Verification items for this drawing (mm, ordinates from the low corner). A direction names the side the tool comes from. Give positions to 0.01 mm unless a question says otherwise; leave off trailing zeros. Loops run counter-clockwise (first coordinate to the right, second up) from the corner with the lowest first, then second, coordinate; pieces in that order, holes last. Notation, with made-up numbers: (76.25, -4.75) -> (125.25, -4.75) arc R22 cw to (125.25, 4.25) -> close; hole circle Ø9 at (5, -32). An arc over 180 degrees is marked (long way). Answer in a Markdown table with one row per item. Add a question column.
Q1. Gauge pin test, flat ends, axial feed: P1, Ø3, axis at y = 6.5, z = 9.5, coming from the -X side; P2, Ø4, axis at x = 5, z = 15.5, coming from the +Y side; P3, Ø4.5, axis at x = 2, y = 5, coming from the -Z side. Record the tip position at first contact, or that the pin passes through.
Q2. Section check A-A on x = 2. Enter the section's corners in (y, z).
Q3. Set-up check for the marked faces 5, 6, 7 and 8: record each of +Z, -Z, +X, -X, +Y, -Y from which the full face is reachable in a straight line by a thin tool's end or side.
Q4. Section check B-B on z = 25.25. Enter the section's corners in (x, y).
Q5. Material ranges on probe 1 along Y at (x, z) = (10, 7); probe 2 along Z at (x, y) = (2.25, 2.5); probe 3 along Z at (x, y) = (11.5, 9.05), recorded low to high.
Q6. Release check for a two-part mould opening along X. For the marked faces 1, 2, 3 and 4 record: pulls with the +X half, pulls with the -X half, needs draft (parallel to the pull), parting line crosses it, or undercut.
Q7. Section check C-C on z = 4. Enter the section's corners in (x, y), and give its area (3 significant figures).
Q8. Section check D-D on x = 5.5. Enter the section's corners in (y, z).
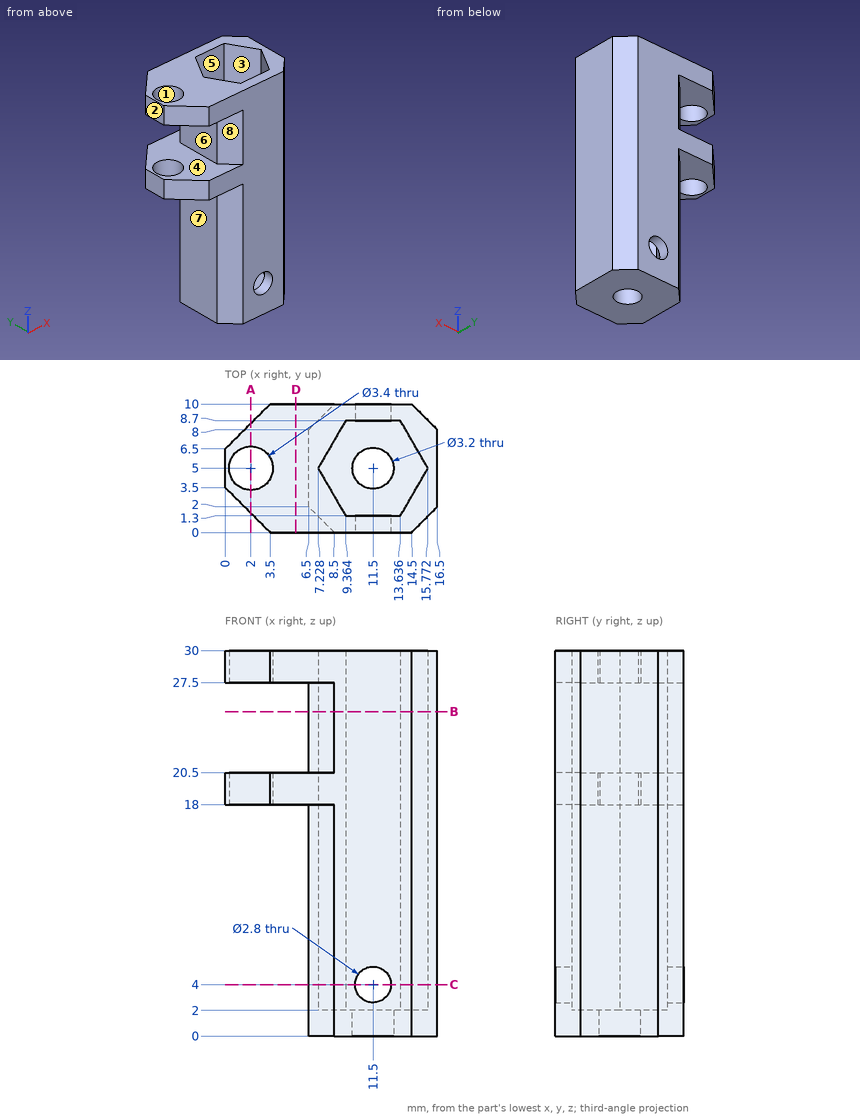
Taken from the geometry:
| question | item | result |
|---|---|---|
| 1 | P1 | stops at x = 6.5 |
| 1 | P2 | stops at y = 8.5 |
| 1 | P3 | stops at z = 18 |
| 2 | outline | (1.5, 18) -> (3.3, 18) -> (3.3, 20.5) -> (1.5, 20.5) -> close; (1.5, 27.5) -> (3.3, 27.5) -> (3.3, 30) -> (1.5, 30) -> close; (6.7, 18) -> (8.5, 18) -> (8.5, 20.5) -> (6.7, 20.5) -> close; (6.7, 27.5) -> (8.5, 27.5) -> (8.5, 30) -> (6.7, 30) -> close |
| 3 | face 5 | +Z |
| 3 | face 6 | -X, +Y, -Y |
| 3 | face 7 | -Z, -X, +Y, -Y |
| 3 | face 8 | -X, -Y |
| 4 | outline | (6.5, 2) -> (8.5, 0) -> (14.5, 0) -> (16.5, 2) -> (16.5, 8) -> (14.5, 10) -> (8.5, 10) -> (6.5, 8) -> close; hole (7.23, 5) -> (9.36, 1.3) -> (13.64, 1.3) -> (15.77, 5) -> (13.64, 8.7) -> (9.36, 8.7) -> close |
| 5 | probe 1 | y = 0 to 1.3, 8.7 to 10 |
| 5 | probe 2 | z = 18 to 20.5, 27.5 to 30 |
| 5 | probe 3 | z = 0 to 2.6, 5.4 to 30 |
| 6 | face 1 | undercut |
| 6 | face 2 | pulls with the -X half |
| 6 | face 3 | undercut |
| 6 | face 4 | needs draft |
| 7 | outline | (6.5, 2) -> (8.5, 0) -> (10.1, 0) -> (10.1, 1.3) -> (9.36, 1.3) -> (7.23, 5) -> (9.36, 8.7) -> (10.1, 8.7) -> (10.1, 10) -> (8.5, 10) -> (6.5, 8) -> close; (12.9, 0) -> (14.5, 0) -> (16.5, 2) -> (16.5, 8) -> (14.5, 10) -> (12.9, 10) -> (12.9, 8.7) -> (13.64, 8.7) -> (15.77, 5) -> (13.64, 1.3) -> (12.9, 1.3) -> close |
| 7 | area | 37.3 mm² |
| 8 | outline | (0, 18) -> (10, 18) -> (10, 20.5) -> (0, 20.5) -> close; (0, 27.5) -> (10, 27.5) -> (10, 30) -> (0, 30) -> close |
